from build123d import *

# Parameters (mm, degrees)
SKETCH1_W           = 65
SKETCH1_H           = 50
SKETCH1_R           = 11
SKETCH1_R_2         = 2
SKETCH1_R_3         = 2.5
BOSS_EXTRUDE1_DEPTH = 5
SKETCH2_R           = 8.5
SKETCH2_R_2         = 4.15
BOSS_EXTRUDE2_DEPTH = 8
FILLET1_R           = 3
CUT_EXTRUDE1_START  = -8
SKETCH3_R           = 4.15
CUT_EXTRUDE1_DEPTH  = 8
FILLET2_R           = 2


with BuildPart() as part:
    # Sketch1 → Boss-Extrude1 (new body)
    with BuildSketch(Plane(origin=(0, 0, 0), x_dir=(1, 0, 0), z_dir=(0, 1, 0))):
        Rectangle(SKETCH1_W, SKETCH1_H)
        with Locations(Location((0, 0, 0), (0, 0, 270))):
            Circle(SKETCH1_R, mode=Mode.SUBTRACT)
        with Locations(Location((15.5, 15.5, 0), (0, 0, 270))):
            Circle(SKETCH1_R_2, mode=Mode.SUBTRACT)
        with Locations(Location((-15.5, 15.5, 0), (0, 0, 270))):
            Circle(SKETCH1_R_2, mode=Mode.SUBTRACT)
        with Locations(Location((15.5, -15.5, 0), (0, 0, 270))):
            Circle(SKETCH1_R_2, mode=Mode.SUBTRACT)
        with Locations(Location((-15.5, -15.5, 0), (0, 0, 270))):
            Circle(SKETCH1_R_2, mode=Mode.SUBTRACT)
        with Locations(Location((26, 20, 0), (0, 0, 270))):
            Circle(SKETCH1_R_3, mode=Mode.SUBTRACT)
        with Locations(Location((-26, 20, 0), (0, 0, 270))):
            Circle(SKETCH1_R_3, mode=Mode.SUBTRACT)
        with Locations(Location((-26, -20, 0), (0, 0, 270))):
            Circle(SKETCH1_R_3, mode=Mode.SUBTRACT)
        with Locations(Location((26, -20, 0), (0, 0, 270))):
            Circle(SKETCH1_R_3, mode=Mode.SUBTRACT)
    extrude(amount=BOSS_EXTRUDE1_DEPTH)

    # Sketch2 → Boss-Extrude2 (add)
    # profile 1 of 2: a face of its own
    with BuildSketch(Plane(origin=(0, 5, 0), x_dir=(1, 0, 0), z_dir=(0, 1, 0))):
        with Locations(Location((22, 0, 0), (0, 0, 270))):
            Circle(SKETCH2_R)
        with Locations(Location((22, 0, 0), (0, 0, 270))):
            Circle(SKETCH2_R_2, mode=Mode.SUBTRACT)
    # profile 2 of 2: a face of its own
    with BuildSketch(Plane(origin=(0, 5, 0), x_dir=(1, 0, 0), z_dir=(0, 1, 0))):
        with Locations(Location((-22, 0, 0), (0, 0, 90))):
            Circle(SKETCH2_R)
        with Locations(Location((-22, 0, 0), (0, 0, 90))):
            Circle(SKETCH2_R_2, mode=Mode.SUBTRACT)
    extrude(amount=BOSS_EXTRUDE2_DEPTH)

    # Fillet1
    fillet1_edges = [part.edges().sort_by_distance(p)[0] for p in [
        (32.5, 2.5, 25),
        (-32.5, 2.5, 25),
        (-32.5, 2.5, -25),
        (32.5, 2.5, -25),
    ]]
    fillet(fillet1_edges, radius=FILLET1_R)

    # Sketch3 → Cut-Extrude1 (cut)
    with BuildSketch(Plane(origin=(0, 5, 0), x_dir=(1, 0, 0), z_dir=(0, 1, 0)).offset(CUT_EXTRUDE1_START)):
        with Locations(Location((-22, 0, 0), (0, 0, 90))):
            Circle(SKETCH3_R)
        with Locations(Location((22, 0, 0), (0, 0, 270))):
            Circle(SKETCH3_R)
    extrude(amount=CUT_EXTRUDE1_DEPTH, mode=Mode.SUBTRACT)

    # Fillet2
    fillet2_edges = [part.edges().sort_by_distance(p)[0] for p in [
        (22, 5, -8.5),
        (-22, 5, 8.5),
    ]]
    fillet(fillet2_edges, radius=FILLET2_R - 0.0001)  # a hair under: the kernel refuses the full size


solid = part.part
Source: CAD feature listing. Evaluate the final solid. Frame: model axes, mm. A direction names the side the tool comes from. Give positions to 0.01 mm unless a question says otherwise; leave off trailing zeros. Order: outer loops, then holes, each group sorted by start corner. A loop starts at its lowest first (then second) coordinate and runs counter-clockwise, first axis right, second up. Notation, with made-up numbers: (-39.75, -20.75) -> (-7.75, -20.75) arc R23 ccw to (-7.75, -10.75) -> close; hole circle Ø3 at (1, 7.5). An arc over 180 degrees is marked (long way). Write item = value, one per line.
Q1. Cut plane A-A, the plane x = -22. Output: boundary loops of the cut face in (y, z).
Data:
outline = (0, -25) -> (5, -25) -> (5, -10.5) arc R2 cw to (7, -8.5) -> (13, -8.5) -> (13, -4.15) -> (0, -4.15) -> close; (0, 4.15) -> (13, 4.15) -> (13, 8.5) -> (7, 8.5) arc R2 cw to (5, 10.5) -> (5, 25) -> (0, 25) -> close
Q2. Cut plane B-B, the plane y = 1. State how many separate pieces and enclosed holes the cut face has, and give its area (3 significant figures).
Data:
separate_pieces = 1
enclosed_holes = 11
area = 2,630 mm^2
Q3. Cut plane C-C, the plane z = 15.5. Output: boundary loops of the cut face in (x, y).
Data:
outline = (-32.5, 0) -> (-17.5, 0) -> (-17.5, 5) -> (-32.5, 5) -> close; (-13.5, 0) -> (13.5, 0) -> (13.5, 5) -> (-13.5, 5) -> close; (17.5, 0) -> (32.5, 0) -> (32.5, 5) -> (17.5, 5) -> close
Q4. Pull-direction query (X, two-part tool) for faces 3 (the face through (31.6, 2.54, 24.14)), 4 (the face through (-31.64, 2.54, -24.1)), 5 (the face through (27.69, 2.46, 18.16)), 6 (the face through (-24.31, 2.46, 18.16)); classes: released by +X, released by -X, zero draft, split by the parting line, or undercut.
Data:
face_3 = released by +X
face_4 = released by -X
face_5 = undercut
face_6 = undercut
Q5. Cut plane D-D, the plane y = 10.25. Output: boundary loops of the cut face in (x, z).
Data:
outline = circle Ø17 at (-22, 0); circle Ø17 at (22, 0); hole circle Ø8.3 at (-22, 0); hole circle Ø8.3 at (22, 0)
Q6. Set-up query: faces 1 (the face through (17.483, 2.465, -15.76)), 2 (the face through (-13.7, 9.96, 1.84)). Return all of +Z, -Z, +X, -X, +Y, -Y with unobstructed straight access to the full face (end or side cutting, diameter ignored); none if empty.
Data:
face_1 = +Y, -Y
face_2 = +Y
Q7. Material intervals for line 1 (X direction, y = 2.65, z = -15.5); line 2 (X direction, y = 2.5, z = -20); line 3 (Z direction, x = -7, y = 2.5), sorted ascending. Write a range as from..to.
Data:
line_1 = -32.5..-17.5, -13.5..13.5, 17.5..32.5
line_2 = -32.5..-28.5, -23.5..23.5, 28.5..32.5
line_3 = -25..-8.49, 8.49..25
Q8. Pin query (flat end, axial travel): pin 1 (3 mm diameter, centred on x = 26, z = 20, fed in from -Y); pin 2 (15 mm diameter, centred on x = 6, z = 10.5, fed in from +Y); pin 3 (2 mm diameter, centred on x = 14, z = 16.5, fed in from -Y). Return the tip coordinate at first contact, or that it passes through.
Data:
pin_1 = through
pin_2 = 5
pin_3 = 0
